Answer from the drawing. Dimensions are ordinates in mm from the lowest x, y and z of the part. A direction names the side the tool comes from. Round coordinates to 2 decimals unless told otherwise and drop trailing zeros. Write each loop counter-clockwise with the first axis right and the second up, starting at its lowest first coordinate (ties: lowest second). Pieces come first, ordered by that corner, then holes. Notation, with made-up numbers: (-19, 16) - (26, 16) arc R18 ccw to (26, 37) - close; hole circle Ø7 at (27, -24). An arc over 180 degrees is marked (long way). Answer in a Markdown table with one row per item.
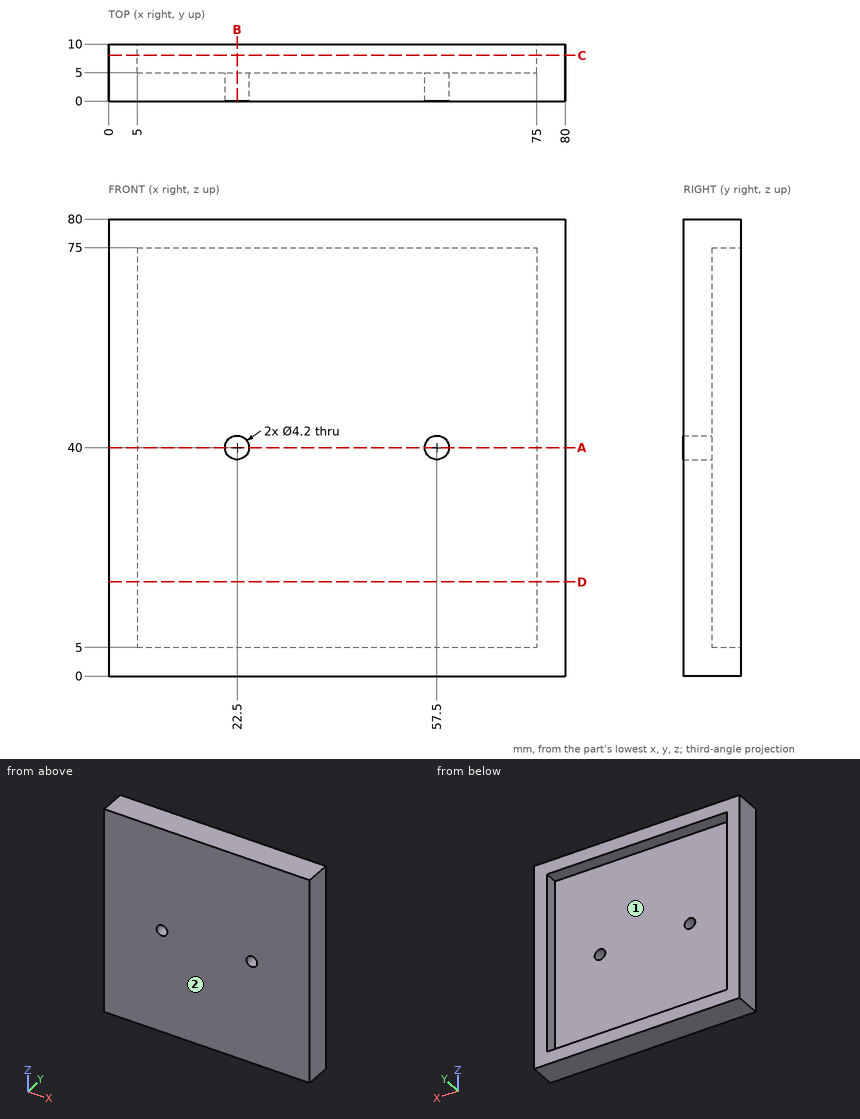
(1) A flat-ended cylindrical pin translates along its axis: pin 1 (1 mm diameter, centred on x = 9, z = 71, fed in from +Y). Find the tip coordinate at first contact, or state that the pin passes through.
Checked values:
| item | result |
|---|---|
| pin 1 | stops at y = 5 |
(2) Section B-B (x = 22.5) is taken. Give the vertices of the cut face in (y, z).
Checked values:
| item | result |
|---|---|
| outline | (0, 0) - (10, 0) - (10, 5) - (5, 5) - (5, 37.9) - (0, 37.9) - close; (0, 42.1) - (5, 42.1) - (5, 75) - (10, 75) - (10, 80) - (0, 80) - close |
(3) Section C-C (y = 8) is taken. Give the vertices of the cut face in (x, z), and give its area (3 significant figures).
Checked values:
| item | result |
|---|---|
| outline | (0, 0) - (80, 0) - (80, 80) - (0, 80) - close; hole (5, 5) - (75, 5) - (75, 75) - (5, 75) - close |
| area | 1,500 mm2 |
(4) Find the intervals of material crossed by line 1 (X direction, y = 1.85, z = 40); line 2 (Z direction, x = 22.5, y = 2.6); line 3 (X direction, y = 8.75, z = 16.5), in increasing order.
Checked values:
| item | result |
|---|---|
| line 1 | x = 0 to 20.4, 24.6 to 55.4, 59.6 to 80 |
| line 2 | z = 0 to 37.9, 42.1 to 80 |
| line 3 | x = 0 to 5, 75 to 80 |
(5) For the marked faces 1 and 2, determine the directions among +Z, -Z, +X, -X, +Y, -Y from which every point of the face is accessible in a straight line to the end or side of a thin tool.
Checked values:
| item | result |
|---|---|
| face 1 | +Y |
| face 2 | +Z, -Z, +X, -X, -Y |
(6) Section A-A (z = 40) is taken. Give the vertices of the cut face in (x, y), and give its area (3 significant figures).
Checked values:
| item | result |
|---|---|
| outline | (0, 0) - (20.4, 0) - (20.4, 5) - (5, 5) - (5, 10) - (0, 10) - close; (24.6, 0) - (55.4, 0) - (55.4, 5) - (24.6, 5) - close; (59.6, 0) - (80, 0) - (80, 10) - (75, 10) - (75, 5) - (59.6, 5) - close |
| area | 408 mm2 |
(7) Section D-D (z = 16.5) is taken. Give the vertices of the cut face in (x, y).
Checked values:
| item | result |
|---|---|
| outline | (0, 0) - (80, 0) - (80, 10) - (75, 10) - (75, 5) - (5, 5) - (5, 10) - (0, 10) - close |
